Build history of the part. All positions in model axes, mm. A direction names the side the tool comes from. Round coordinates to 2 decimals unless told otherwise and drop trailing zeros. Loops run counter-clockwise (first coordinate to the right, second up) from the corner with the lowest first, then second, coordinate; pieces in that order, holes last. Notation, with made-up numbers: M 60.5,-14.5 L 85.5,-14.5 A10 ccw 85.5,-5.5 Z; hole C 60,79 d4. An arc over 180 degrees is marked long. Write each question's results on one line, items separated by ' | '. Start each with the question number.
```python
from build123d import *

# Parameters (mm, degrees)
SALIENTE_EXTRUIR1_DEPTH = 19
CROQUIS3_W              = 52.808095268
CROQUIS3_H              = 23.684781413
SALIENTE_EXTRUIR2_DEPTH = 3
CROQUIS4_W              = 12.057899081
CROQUIS4_H              = 3.984349261
CORTAR_EXTRUIR1_DEPTH   = 26
SALIENTE_EXTRUIR3_DEPTH = 3
SALIENTE_EXTRUIR4_DEPTH = 1.3


with BuildPart() as part:
    # Croquis1 → Saliente-Extruir1 (new body)
    with BuildSketch(Plane.XY):
        Polygon((-24.404047634, 20.4), (-24.404047634, -1.284781413), (24.404047634, -1.284781413), (24.404047634, 20.4), (26.404047634, 20.4), (26.404047634, -3.284781413), (-26.404047634, -3.284781413), (-26.404047634, 20.4), align=None)
    extrude(amount=-SALIENTE_EXTRUIR1_DEPTH)

    # Croquis3 → Saliente-Extruir2 (add)
    with BuildSketch(Plane(origin=(0, 0, -19), x_dir=(-1, 0, 0), z_dir=(0, 0, -1))):
        with Locations((0, 8.557609294)):
            Rectangle(CROQUIS3_W, CROQUIS3_H)
    extrude(amount=SALIENTE_EXTRUIR2_DEPTH)

    # Croquis4 → Cortar-Extruir1 (cut)
    with BuildSketch(Plane.XZ.offset(3.284781413)):
        with Locations((-0.283990929, -18.525322076)):
            Rectangle(CROQUIS4_W, CROQUIS4_H)
    extrude(amount=-CORTAR_EXTRUIR1_DEPTH, mode=Mode.SUBTRACT)

    # Croquis8 → Saliente-Extruir3 (add)
    with BuildSketch(Plane(origin=(0, -1.284781413, 0), x_dir=(1, 0, 0), z_dir=(0, 1, 0))):
        with BuildLine():
            Line((-20.273206473, 1.311556937), (-18.273206473, 1.311556937))
            ThreePointArc((-18.273206473, 1.311556937), (-17.806113325, 1.427348822), (-17.447191369, 1.747908954))
            Line((-17.447191369, 1.747908954), (-20.273206473, 8.311556937))
            ThreePointArc((-20.273206473, 8.311556937), (-20.980313254, 8.018663718), (-21.273206473, 7.311556937))
            Line((-21.273206473, 7.311556937), (-21.273206473, 2.311556937))
            ThreePointArc((-21.273206473, 2.311556937), (-20.980313254, 1.604450156), (-20.273206473, 1.311556937))
        make_face()
        with BuildLine():
            Line((20.273206473, 1.311556937), (18.273206473, 1.311556937))
            ThreePointArc((18.273206473, 1.311556937), (17.806113325, 1.427348822), (17.447191369, 1.747908954))
            Line((17.447191369, 1.747908954), (20.273206473, 8.311556937))
            ThreePointArc((20.273206473, 8.311556937), (20.980313254, 8.018663718), (21.273206473, 7.311556937))
            Line((21.273206473, 7.311556937), (21.273206473, 2.311556937))
            ThreePointArc((21.273206473, 2.311556937), (20.980313254, 1.604450156), (20.273206473, 1.311556937))
        make_face()
    extrude(amount=SALIENTE_EXTRUIR3_DEPTH)

    # Croquis9 → Saliente-Extruir4 (add)
    with BuildSketch(Plane(origin=(0, 0, -9.5), x_dir=(-1, 0, 0), z_dir=(0, 0, -1))):
        with BuildLine():
            Line((24.404047634, -1.284781413), (13.491213659, -1.284781413))
            add(Edge.make_bspline(
                [(24.404047634, 8.114982057), (20.954967317, 0.215218587), (13.491213659, -1.284781413)],
                knots=[0, 0, 0, 1, 1, 1], degree=2))
            Line((24.404047634, 8.114982057), (24.404047634, -1.284781413))
        make_face()
        with BuildLine():
            Line((-24.404047634, -1.284781413), (-13.491213659, -1.284781413))
            add(Edge.make_bspline(
                [(-24.404047634, 8.114982057), (-20.954967317, 0.215218587), (-13.491213659, -1.284781413)],
                knots=[0, 0, 0, 1, 1, 1], degree=2))
            Line((-24.404047634, 8.114982057), (-24.404047634, -1.284781413))
        make_face()
    extrude(amount=SALIENTE_EXTRUIR4_DEPTH)


solid = part.part
```
Item 1: Saw through at B-B, the plane x = -4.5. Give the cut face in (y, z), then the cut area to 3 significant figures.
Item 2: Saw through at C-C, the plane y = 18. Give the cut face in (x, z).
Item 3: Saw through at D-D, the plane x = 12. Give the cut face in (y, z), then the cut area to 3 significant figures.
Item 4: Drop flat-ended pins along their axis: pin 1 (9 mm diameter, centred on x = -18, y = 6.5, fed in from +Z); pin 2 (8 mm diameter, centred on x = 3.5, z = -13.5, fed in from +Y); pin 3 (4 mm diameter, centred on x = 19.5, z = -5.5, fed in from +Y). Give the stop position or say it passes through.
Item 5: Saw through at A-A, the plane z = -17.75. Give the cut face in (x, y), then the cut area to 3 significant figures.
Item 6: Mould opens along X. For faces 4 (the flat face through (0, -2, 0)), 5 (the flat face through (26.404, 8, -11)), 6 (the flat face through (-21.273, 0, -5)) say: released by +X, released by -X, zero draft, split by the parting line, or undercut.
Item 7: Tool access for faces 1 (the cylindrical face through (-20.988, 0.194, -1.612)), 2 (the flat face through (5.745, 5.8, -19.4)), 3 (the flat face through (22, 1, -9.5)): list every direction of +Z, -Z, +X, -X, +Y, -Y with a clear straight run to the whole face (end or side of a thin tool).
Item 8: Drill centre lines: line 1 along X through (y, z) = (12.25, -10); line 2 along X through (y, z) = (1.75, -19.5); line 3 along Z through (x, y) = (-22.5, -0.5). Where is each one in solid material? Low to high. Write a range as [from, to].
Working result:
1) outline: M -3.28,-22 L 20.4,-22 L 20.4,-20.52 L -3.28,-20.52 Z; M -3.28,-16.53 L -1.28,-16.53 L -1.28,0 L -3.28,0 Z | area: 68.2 mm²
2) outline: M -26.4,-22 L 26.4,-22 L 26.4,0 L 24.4,0 L 24.4,-19 L 5.74,-19 L 5.74,-20.52 L -6.31,-20.52 L -6.31,-19 L -24.4,-19 L -24.4,0 L -26.4,0 Z
3) outline: M -3.28,-22 L 20.4,-22 L 20.4,-19 L -1.28,-19 L -1.28,0 L -3.28,0 Z | area: 109 mm²
4) pin 1: stops at z = -19 | pin 2: stops at y = -1.28 | pin 3: stops at y = 1.72
5) outline: M -26.4,-3.28 L -6.31,-3.28 L -6.31,-1.28 L -24.4,-1.28 L -24.4,20.4 L -26.4,20.4 Z; M 5.74,-3.28 L 26.4,-3.28 L 26.4,20.4 L 24.4,20.4 L 24.4,-1.28 L 5.74,-1.28 Z | area: 168 mm²
6) face 4: zero draft | face 5: released by +X | face 6: undercut
7) face 1: +Z, +Y | face 2: +Y, -Y | face 3: +Y
8) line 1: x = [-26.4, -24.4], [24.4, 26.4] | line 2: x = [-26.4, -6.31], [5.74, 26.4] | line 3: z = [-22, -19], [-10.8, -9.5]
